Source: three-view drawing plus pictorial views. Frame: mm from the lowest corner of the part. Give positions to 0.01 mm unless a question says otherwise; leave off trailing zeros. Order: outer loops, then holes, each group sorted by start corner. A loop starts at its lowest first (then second) coordinate and runs counter-clockwise, first axis right, second up. Notation, with made-up numbers: (59.5, -32) - (63.5, -32) arc R19 ccw to (63.5, 3) - close; hole circle Ø2 at (-0.75, 12.25). An arc over 180 degrees is marked (long way). Answer in a Markdown table with one row per item. Add a question column.
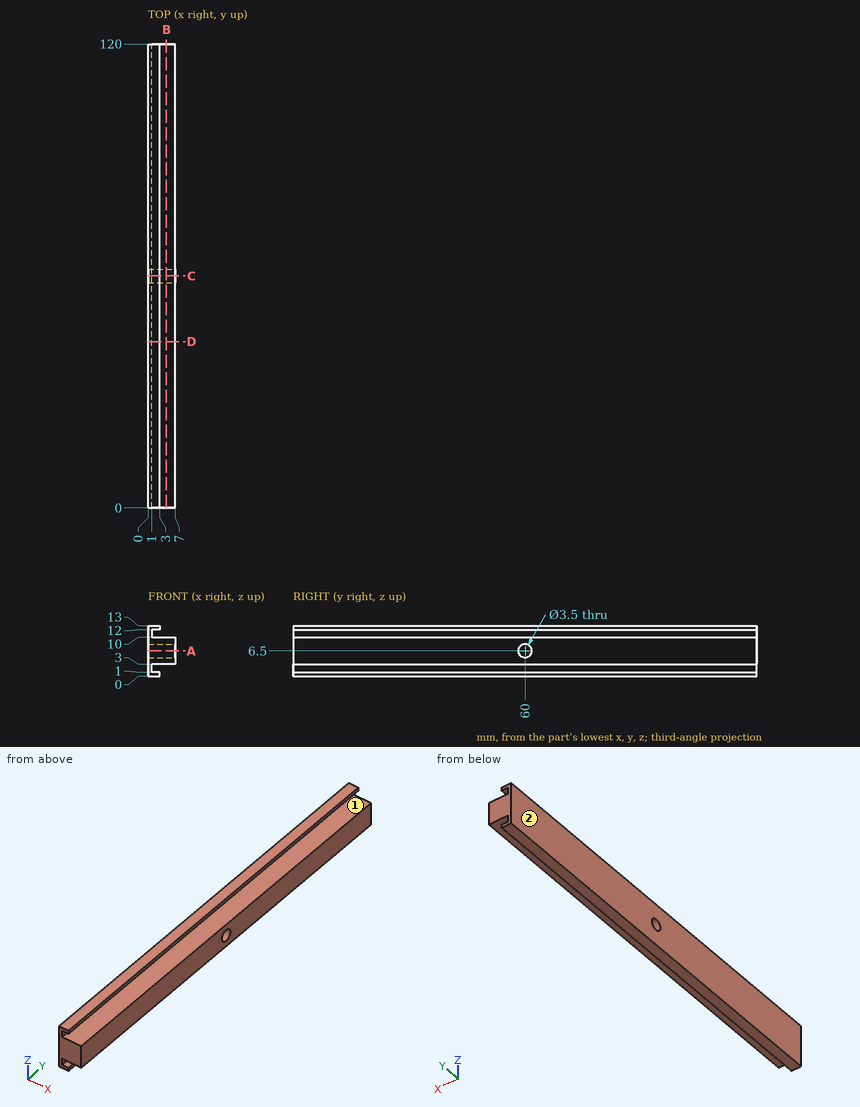
Q1. Section B-B, the plane x = 4.75. Return loops of the section in (y, z).
Q2. Section C-C, the plane y = 60. Return loops of the section in (x, z), then the cut area to 3 significant figures.
Q3. Section D-D, the plane y = 43. Return loops of the section in (x, z).
Q4. Pull-direction query (Z, two-part tool) for the marked faces 1 and 2; classes: +Z half, -Z half, draft (parallel to the pull), parting line (faces both ways), or undercut.
Q5. Contact query for flat-ended pins moving along their axis: P1, Ø0.6, axis at y = 59.5, z = 11.5, coming from the +X side; P2, Ø1.1, axis at y = 32, z = 12.5, coming from the +X side. Output: stop coordinate, or through.
Q6. Line query: probe 1 along Z at (x, y) = (1.5, 107.5); probe 2 along Z at (x, y) = (2.5, 60); probe 3 along Y at (x, z) = (1.75, 6.5). Output: solid intervals per line, ascending.
Q7. Section A-A, the plane z = 6.5. Return loops of the section in (x, y), then the cut area to 4 significant figures.
Computed:
| question | item | result |
|---|---|---|
| 1 | outline | (0, 3) - (120, 3) - (120, 10) - (0, 10) - close; hole circle Ø3.5 at (60, 6.5) |
| 2 | outline | (0, 0) - (3, 0) - (3, 1) - (1, 1) - (1, 3) - (7, 3) - (7, 4.75) - (0, 4.75) - close; (0, 8.25) - (7, 8.25) - (7, 10) - (1, 10) - (1, 12) - (3, 12) - (3, 13) - (0, 13) - close |
| 2 | area | 34.5 mm^2 |
| 3 | outline | (0, 0) - (3, 0) - (3, 1) - (1, 1) - (1, 3) - (7, 3) - (7, 10) - (1, 10) - (1, 12) - (3, 12) - (3, 13) - (0, 13) - close |
| 4 | face 1 | undercut |
| 4 | face 2 | draft |
| 5 | P1 | stops at x = 1 |
| 5 | P2 | stops at x = 3 |
| 6 | probe 1 | z = 0 to 1, 3 to 10, 12 to 13 |
| 6 | probe 2 | z = 0 to 1, 3 to 4.75, 8.25 to 10, 12 to 13 |
| 6 | probe 3 | y = 0 to 58.25, 61.75 to 120 |
| 7 | outline | (0, 0) - (7, 0) - (7, 58.25) - (0, 58.25) - close; (0, 61.75) - (7, 61.75) - (7, 120) - (0, 120) - close |
| 7 | area | 815.5 mm^2 |
